from build123d import *

# Parameters (mm, degrees)
ESQUISSE1_R             = 1.5
BOSS_EXTRU_1_DEPTH      = 4
ESQUISSE1_4_R           = 1.5
ENL_V_MAT_EXTRU_1_DEPTH = 2


with BuildPart() as part:
    # Esquisse1 → Boss.-Extru.1 (new body)
    with BuildSketch(Plane.XY):
        with BuildLine():
            Line((0, 3), (25, 3))
            ThreePointArc((25, 3), (28, 0), (25, -3))
            Line((25, -3), (0, -3))
            ThreePointArc((0, -3), (-3, 0), (0, 3))
        make_face()
        Circle(ESQUISSE1_R, mode=Mode.SUBTRACT)
        with Locations((25, 0)):
            Circle(ESQUISSE1_R, mode=Mode.SUBTRACT)
    extrude(amount=BOSS_EXTRU_1_DEPTH)

    # Esquisse1_4 → Enl_v. mat.-Extru.1 (cut)
    with BuildSketch(Plane.XY):
        with BuildLine():
            Line((0, 3), (25, 3))
            ThreePointArc((25, 3), (28, 0), (25, -3))
            Line((25, -3), (0, -3))
            ThreePointArc((0, -3), (-3, 0), (0, 3))
        make_face()
        Circle(ESQUISSE1_4_R, mode=Mode.SUBTRACT)
        with Locations((25, 0)):
            Circle(ESQUISSE1_4_R, mode=Mode.SUBTRACT)
    extrude(amount=ENL_V_MAT_EXTRU_1_DEPTH, mode=Mode.SUBTRACT)


solid = part.part
Read the model definition and answer for the solid it produces. Units are mm, in the model's axes. Round coordinates to 2 decimals unless told otherwise and drop trailing zeros. Loops run counter-clockwise (first coordinate to the right, second up) from the corner with the lowest first, then second, coordinate; pieces in that order, holes last.
Q1. Section C-C on y = 2.2 is taken. Write down the section's boundary in (x, z).
Q2. Section A-A on y = 0 is taken. Write down the section's boundary in (x, z), and give its area (3 significant figures).
Q3. Determine the mould class of faces 1 (the face through (28, 0, 3)), 2 (the face through (12, 3, 3)), 3 (the face through (23.5, 0.07, 2.99)) for opening direction X: released by +X, released by -X, zero draft, split by the parting line, or undercut.
Q4. Consider probe 1 along Y at (x, z) = (0, 2.55); probe 2 along X at (y, z) = (-1.15, 3.05); probe 3 along X at (y, z) = (1, 3.3). Determine where each line is inside the solid, lowest interval first.
Q5. Section D-D on y = -2.25 is taken. Write down the section's boundary in (x, z), and give its area (3 significant figures).
Q6. Section B-B on z = 3.25 is taken. Write down the section's boundary in (x, y), and give its area (3 significant figures).
Output:
1. outline: (-2.04, 2) - (27.04, 2) - (27.04, 4) - (-2.04, 4) - close
2. outline: (-3, 2) - (-1.5, 2) - (-1.5, 4) - (-3, 4) - close; (1.5, 2) - (23.5, 2) - (23.5, 4) - (1.5, 4) - close; (26.5, 2) - (28, 2) - (28, 4) - (26.5, 4) - close
2. area: 50.0 mm2
3. face 1: released by +X
3. face 2: zero draft
3. face 3: undercut
4. probe 1: y = -3 to -1.5, 1.5 to 3
4. probe 2: x = -2.77 to -0.96, 0.96 to 24.04, 25.96 to 27.77
4. probe 3: x = -2.83 to -1.12, 1.12 to 23.88, 26.12 to 27.83
5. outline: (-1.98, 2) - (26.98, 2) - (26.98, 4) - (-1.98, 4) - close
5. area: 57.9 mm2
6. outline: (0, -3) - (25, -3) arc R3 ccw to (25, 3) - (0, 3) arc R3 ccw to start; hole circle Ø3 at (0, 0); hole circle Ø3 at (25, 0)
6. area: 164 mm2
